from build123d import *

# Parameters (mm, degrees)
F0_W     = 368.3
F0_H     = 177.8
F1_DEPTH = 25.4
F2_W     = 97.073552
F2_H     = 88.9
F3_DEPTH = 368.3


with BuildPart() as f1:
    # F0 (on Front) → F1 (new body)
    with BuildSketch(Plane.XZ):
        with Locations((184.15, -88.9)):
            Rectangle(F0_W, F0_H)
    extrude(amount=F1_DEPTH)

    # F2 (on Right) → F3 (cut)
    with BuildSketch(Plane.YZ):
        with Locations((-60.2259, -44.45)):
            Rectangle(F2_W, F2_H)
    extrude(amount=F3_DEPTH, mode=Mode.SUBTRACT)


solid = f1.part
CAD build for the part. Positions are in the model's coordinates, mm. A direction names the side the tool comes from. Give positions to 0.01 mm unless a question says otherwise; leave off trailing zeros. Write each loop counter-clockwise with the first axis right and the second up, starting at its lowest first coordinate (ties: lowest second). Pieces come first, ordered by that corner, then holes. Notation, with made-up numbers: (49.5, 0) - (98.5, 0) arc R18 ccw to (98.5, 23) - close; hole circle Ø3 at (32, 22.5). An arc over 180 degrees is marked (long way). Put each result on its own line as item: value.
(1) Saw through at C-C (y = -22). List the corners of the cut face in (x, z).
Working result:
outline: (0, -177.8) - (368.3, -177.8) - (368.3, -88.9) - (0, -88.9) - close
(2) Saw through at B-B (z = -41). List the corners of the cut face in (x, y).
Working result:
outline: (0, -11.69) - (368.3, -11.69) - (368.3, 0) - (0, 0) - close
(3) Tool access for faces 1 (the flat face through (182, 0, -88)), 2 (the flat face through (182, -19, -88.9)): list every direction of +Z, -Z, +X, -X, +Y, -Y with a clear straight run to the whole face (end or side of a thin tool).
Working result:
face 1: +Z, -Z, +X, -X, +Y
face 2: +Z, +X, -X, -Y
(4) Saw through at A-A (x = 107). List the corners of the cut face in (y, z).
Working result:
outline: (-25.4, -177.8) - (0, -177.8) - (0, 0) - (-11.69, 0) - (-11.69, -88.9) - (-25.4, -88.9) - close
(5) Wall check: L1, parallel to Z at x = 205, y = -22.75; L2, parallel to Y at x = 310.5, z = -81. Give the ranges that are in metal, low to high.
Working result:
L1: -177.8 to -88.9
L2: -11.69 to 0
(6) Drop a flat-ended pin along its axis: pin 1 Ø4 at (x, y) = (257.5, -18) entering from +Z. Give the stop position or say it passes through.
Working result:
pin 1: z = -88.9
